Model file for the job. Use its own axes, mm. Round coordinates to 2 decimals unless told otherwise and drop trailing zeros. Order: outer loops, then holes, each group sorted by start corner. A loop starts at its lowest first (then second) coordinate and runs counter-clockwise, first axis right, second up. Notation, with made-up numbers: (32, 17) - (55, 17) arc R10 ccw to (55, 28) - close; hole circle Ø9 at (5.5, 19). An arc over 180 degrees is marked (long way). Answer as CSV lines item,"result". Start each with the question number.
1. Band-saw the part on C-C on y = -5. List the corners of the cut face in (x, z), then the cut area to 3 significant figures.
2. Pin check, flat tips, straight feed: pin 1 Ø6 at (y, z) = (-5, 0) entering from +X; pin 2 Ø3 at (x, y) = (0, -5) entering from +Z; pin 3 Ø2 at (x, y) = (29.5, -5.5) entering from +Z; pin 4 Ø4.5 at (x, y) = (30, -4.5) entering from -Z. Stop position of each tip, or through.
3. Band-saw the part on B-B on z = 0. List the corners of the cut face in (x, y), then the cut area to 3 significant figures.
4. Band-saw the part on A-A on x = 0. List the corners of the cut face in (y, z), then the cut area to 3 significant figures.
5. Wall check: line 1 along X through (y, z) = (-5, -4); line 2 along Z through (x, y) = (66.5, -5); line 3 along Z through (x, y) = (-43, -5). Give the ranges that are in metal, low to high. Write a range as [from, to].
6. Band-saw the part on D-D on x = -47.5. List the corners of the cut face in (y, z).
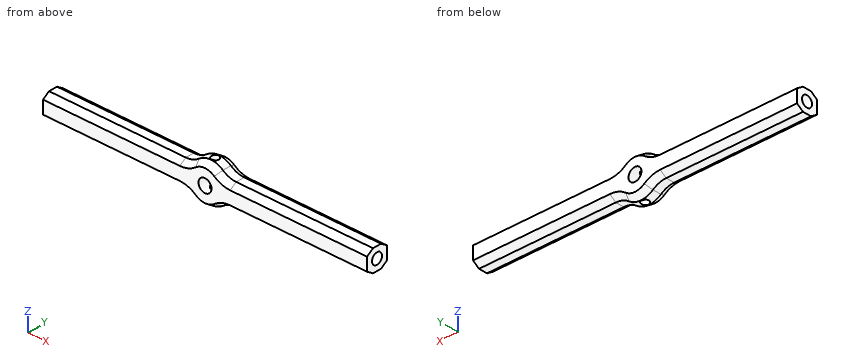
```python
from build123d import *

# Parameters (mm, degrees)
F0_R          = 3
F1_DEPTH      = 10
F2_R          = 2.5
F3_DEPTH      = 25
F4_R          = 1.75
F5_DEPTH      = 9.001
F5_DEPTH_BACK = 9.001
F6_R          = 10
F7_SIZE2      = 3
F7_SIZE       = 2
F7_2_SIZE2    = 3
F7_2_SIZE     = 2


# Not quite as in the source:
# - a pattern or mirror of a feature is missing from the dataset's text; its kind, count and spacing are read off the source's solid


with BuildPart() as f1:
    # F0 (on Front) → F1 (new body)
    with BuildSketch(Plane.XZ):
        with BuildLine():
            Line((75, 5), (7.4833147735, 5))
            ThreePointArc((7.4833147735, 5), (0, 9), (-7.4833147735, 5))
            Line((-7.4833147735, 5), (-75, 5))
            Line((-75, 5), (-75, -5))
            Line((-75, -5), (-7.4833147735, -5))
            ThreePointArc((-7.4833147735, -5), (0, -9), (7.4833147735, -5))
            Line((7.4833147735, -5), (75, -5))
            Line((75, -5), (75, 5))
        make_face()
        Circle(F0_R, mode=Mode.SUBTRACT)
    extrude(amount=F1_DEPTH)

    # F2 (on face) → F3 (cut)
    with BuildSketch(Plane(origin=(-75, 0, 0), x_dir=(0, -1, 0), z_dir=(-1, 0, 0))):
        with Locations((5, 0)):
            Circle(F2_R)
    f3 = extrude(amount=-F3_DEPTH, mode=Mode.SUBTRACT)

    # F3_copies: F3 across plane
    add(f3.mirror(Plane(origin=(0, 0, 0), x_dir=(0, 0, 1), z_dir=(1, 0, 0))), mode=Mode.SUBTRACT)

    # F4 (on Top) → F5 (cut, two sides)
    with BuildSketch(Plane.XY) as f5_sk:
        with Locations((0, -5)):
            Circle(F4_R)
    extrude(amount=-F5_DEPTH, mode=Mode.SUBTRACT)
    extrude(f5_sk.sketch, amount=F5_DEPTH_BACK, mode=Mode.SUBTRACT)

    # F6
    f6_edges = [f1.edges().sort_by_distance(p)[0] for p in [
        (-7.483315, -5, 5),
        (7.483315, -5, 5),
        (7.483315, -5, -5),
        (-7.483315, -5, -5),
    ]]
    fillet(f6_edges, radius=F6_R)

    # F7
    f7_edges = [f1.edges().sort_by_distance(p)[0] for p in [
        (-43.330952, -10, 5),
        (-43.330952, -10, -5),
    ]]
    f7_side = f1.faces().sort_by_distance((43.330952, -10, -3.489239))[0]
    chamfer(f7_edges, length=F7_SIZE, length2=F7_SIZE2, reference=f7_side)

    # F7#2
    f7_2_edges = [f1.edges().sort_by_distance(p)[0] for p in [
        (-43.330952, 0, 5),
        (-43.330952, 0, -5),
    ]]
    f7_2_side = f1.faces().sort_by_distance((43.330952, 0, -3.489239))[0]
    chamfer(f7_2_edges, length=F7_2_SIZE, length2=F7_2_SIZE2, reference=f7_2_side)


solid = f1.part
```
Reply:
1,outline,"(-75, -5) - (-11.66, -5) arc R10 cw to (-5.52, -7.11) arc R9 ccw to (-1.75, -8.83) - (-1.75, -2.44) arc R3 cw to (-1.75, 2.44) - (-1.75, 8.83) arc R9 ccw to (-5.52, 7.11) arc R10 cw to (-11.66, 5) - (-75, 5) - (-75, 2.5) - (-50, 2.5) - (-50, -2.5) - (-75, -2.5) - close; (1.75, -8.83) arc R9 ccw to (5.52, -7.11) arc R10 cw to (11.66, -5) - (75, -5) - (75, -2.5) - (50, -2.5) - (50, 2.5) - (75, 2.5) - (75, 5) - (11.66, 5) arc R10 cw to (5.52, 7.11) arc R9 ccw to (1.75, 8.83) - (1.75, 2.44) arc R3 cw to (1.75, -2.44) - close"
1,area,"1,270 mm2"
2,pin 1,"stops at x = 75"
2,pin 2,"passes through"
2,pin 3,"stops at z = 5"
2,pin 4,"stops at z = -5"
3,outline,"(-75, -10) - (-3, -10) - (-3, 0) - (-75, 0) - (-75, -2.5) - (-50, -2.5) - (-50, -7.5) - (-75, -7.5) - close; (3, -10) - (75, -10) - (75, -7.5) - (50, -7.5) - (50, -2.5) - (75, -2.5) - (75, 0) - (3, 0) - close"
3,area,"1,190 mm2"
4,outline,"(-10, -7) - (-7, -9) - (-6.75, -9) - (-6.75, -3) - (-10, -3) - close; (-10, 3) - (-6.75, 3) - (-6.75, 9) - (-7, 9) - (-10, 7) - close; (-3.25, -9) - (-3, -9) - (0, -7) - (0, -3) - (-3.25, -3) - close; (-3.25, 3) - (0, 3) - (0, 7) - (-3, 9) - (-3.25, 9) - close"
4,area,"66.0 mm2"
5,line 1,"x = [-75, -1.75], [1.75, 75]"
5,line 2,"z = [-5, -2.5], [2.5, 5]"
5,line 3,"z = [-5, 5]"
6,outline,"(-10, -3) - (-7, -5) - (-3, -5) - (0, -3) - (0, 3) - (-3, 5) - (-7, 5) - (-10, 3) - close"
